from build123d import *

# Parameters (mm, degrees)
SKETCH1_W           = 180
SKETCH1_H           = 2
BOSS_EXTRUDE1_DEPTH = 20
SKETCH2_R           = 3
CUT_EXTRUDE1_DEPTH  = 20
CUT_EXTRUDE2_DEPTH  = 20


with BuildPart() as part:
    # Sketch1 → Boss-Extrude1 (new body)
    with BuildSketch(Plane.XY):
        Rectangle(SKETCH1_W, SKETCH1_H)
    extrude(amount=BOSS_EXTRUDE1_DEPTH)

    # Sketch2 → Cut-Extrude1 (cut)
    with BuildSketch(Plane(origin=(0, 1, 0), x_dir=(1, 0, 0), z_dir=(0, 1, 0))):
        with Locations(Location((82, -10, 0), (0, 0, 270))):
            Circle(SKETCH2_R)
        with Locations(Location((-82, -10, 0), (0, 0, 180))):
            Circle(SKETCH2_R)
    extrude(amount=-CUT_EXTRUDE1_DEPTH, mode=Mode.SUBTRACT)

    # Sketch3 → Cut-Extrude2 (cut)
    with BuildSketch(Plane(origin=(0, 1, 0), x_dir=(1, 0, 0), z_dir=(0, 1, 0))):
        Polygon((-14, -4), (-10, 0), (-18, 0), align=None)
        Polygon((-22, -4), (-18, 0), (-26, 0), align=None)
        Polygon((82, -4), (86, 0), (78, 0), align=None)
        Polygon((86, 0), (90, -4), (90, 0), align=None)
        Polygon((74, -4), (78, 0), (70, 0), align=None)
        Polygon((66, -4), (70, 0), (62, 0), align=None)
        Polygon((58, -4), (62, 0), (54, 0), align=None)
        Polygon((50, -4), (54, 0), (46, 0), align=None)
        Polygon((42, -4), (46, 0), (38, 0), align=None)
        Polygon((34, -4), (38, 0), (30, 0), align=None)
        Polygon((26, -4), (30, 0), (22, 0), align=None)
        Polygon((18, -4), (22, 0), (14, 0), align=None)
        Polygon((10, -4), (14, 0), (6, 0), align=None)
        Polygon((2, -4), (6, 0), (-2, 0), align=None)
        Polygon((-30, -4), (-26, 0), (-34, 0), align=None)
        Polygon((-6, -4), (-2, 0), (-10, 0), align=None)
        Polygon((-38, -4), (-34, 0), (-42, 0), align=None)
        Polygon((-86, -4), (-82, 0), (-90, 0), align=None)
        Polygon((-78, -4), (-74, 0), (-82, 0), align=None)
        Polygon((-70, -4), (-66, 0), (-74, 0), align=None)
        Polygon((-62, -4), (-58, 0), (-66, 0), align=None)
        Polygon((-54, -4), (-50, 0), (-58, 0), align=None)
        Polygon((-46, -4), (-42, 0), (-50, 0), align=None)
    extrude(amount=-CUT_EXTRUDE2_DEPTH, mode=Mode.SUBTRACT)


solid = part.part
Can you work these out from the model? Positions are in its coordinate system, mm. A direction names the side the tool comes from. Round coordinates to 2 decimals unless told otherwise and drop trailing zeros. Write each loop counter-clockwise with the first axis right and the second up, starting at its lowest first coordinate (ties: lowest second). Pieces come first, ordered by that corner, then holes. Notation, with made-up numbers: (-37, 35.25) -> (-15, 35.25) arc R18 cw to (-15, 65.25) -> close; hole circle Ø6 at (-10, 62). An arc over 180 degrees is marked (long way). Use one line per item in the form item = value. Start each with the question number.
Q1. Imagine slicing it at B-B (y = -0.3). Count the separate pieces of the cut face and the enclosed holes in it, then the cut area to 3 significant figures.
Q2. Which directions (+Z, -Z, +X, -X, +Y, -Y) give clear straight access to the entire face, cutting with the end or side of a thin tool? Please do faces 4 (the face through (-72, 0, 2)), 5 (the face through (88, 0, 2)).
Q3. We'd pull the mould along Z, two halves only. Please class faces 1 (the face through (-1, 1, 10)), 2 (the face through (79.07, 0.01, 9.35)), 3 (the face through (16, 0, 2)): +Z half, -Z half, draft (parallel to the pull), parting line (faces both ways), or undercut.
Q4. If I drill on probe 1 along Z at (x, y) = (-82, 0.2); probe 2 along X at (y, z) = (-0.55, 12); probe 3 along X at (y, z) = (0.7, 12.25), over which ranges is the centre line in solid material (lowest first)? Write a range as [from, to].
Q5. Imagine slicing it at A-A (z = 10). Please give me the cut outline in (x, y).
Worked out:
q1.separate_pieces = 1
q1.enclosed_holes = 2
q1.area = 3,180 mm^2
q2.face_4 = -Z, +Y, -Y
q2.face_5 = -Z, +X, +Y, -Y
q3.face_1 = draft
q3.face_2 = undercut
q3.face_3 = -Z half
q4.probe_1 = [0, 7], [13, 20]
q4.probe_2 = [-90, -84.24], [-79.76, 79.76], [84.24, 90]
q4.probe_3 = [-90, -83.98], [-80.02, 80.02], [83.98, 90]
q5.outline = (-90, -1) -> (-85, -1) -> (-85, 1) -> (-90, 1) -> close; (-79, -1) -> (79, -1) -> (79, 1) -> (-79, 1) -> close; (85, -1) -> (90, -1) -> (90, 1) -> (85, 1) -> close
